from build123d import *

# Parameters (mm, degrees)
SKETCH1_R           = 9.525
SKETCH1_R_2         = 4.445
BOSS_EXTRUDE1_DEPTH = 3.048
SKETCH2_R           = 6.985
SKETCH2_R_2         = 4.445
BOSS_EXTRUDE2_DEPTH = 57.912
SKETCH3_R           = 9.525
SKETCH3_R_2         = 6.985
SKETCH3_R_3         = 4.445
BOSS_EXTRUDE3_DEPTH = 3.048


with BuildPart() as part:
    # Sketch1 → Boss-Extrude1 (new body)
    with BuildSketch(Plane(origin=(0, 0, 0), x_dir=(1, 0, 0), z_dir=(0, 1, 0))):
        with Locations(Location((0, 0, 0), (0, 0, 270))):  # turned: the seam where the file's is
            Circle(SKETCH1_R)
        with Locations(Location((0, 0, 0), (0, 0, 270))):  # turned: the seam where the file's is
            Circle(SKETCH1_R_2, mode=Mode.SUBTRACT)
    extrude(amount=BOSS_EXTRUDE1_DEPTH)

    # Sketch2 → Boss-Extrude2 (add)
    with BuildSketch(Plane(origin=(0, 3.048, 0), x_dir=(1, 0, 0), z_dir=(0, 1, 0))):
        with Locations(Location((0, 0, 0), (0, 0, 270))):  # turned: the seam where the file's is
            Circle(SKETCH2_R)
        with Locations(Location((0, 0, 0), (0, 0, 270))):  # turned: the seam where the file's is
            Circle(SKETCH2_R_2, mode=Mode.SUBTRACT)
    extrude(amount=BOSS_EXTRUDE2_DEPTH)

    # Sketch3 → Boss-Extrude3 (add)
    with BuildSketch(Plane(origin=(0, 60.96, 0), x_dir=(1, 0, 0), z_dir=(0, 1, 0))):
        with Locations(Location((0, 0, 0), (0, 0, 270))):  # turned: the seam where the file's is
            Circle(SKETCH3_R)
        with Locations(Location((0, 0, 0), (0, 0, 270))):  # turned: the seam where the file's is
            Circle(SKETCH3_R_2, mode=Mode.SUBTRACT)
        with Locations(Location((0, 0, 0), (0, 0, 270))):  # turned: the seam where the file's is
            Circle(SKETCH3_R_2)
        with Locations(Location((0, 0, 0), (0, 0, 270))):  # turned: the seam where the file's is
            Circle(SKETCH3_R_3, mode=Mode.SUBTRACT)
    extrude(amount=BOSS_EXTRUDE3_DEPTH)


solid = part.part
Could you check a few things on this model? Use its own coordinates, in mm. A direction names the side the tool comes from. Round coordinates to 2 decimals unless told otherwise and drop trailing zeros. Write each loop counter-clockwise with the first axis right and the second up, starting at its lowest first coordinate (ties: lowest second). Pieces come first, ordered by that corner, then holes. Notation, with made-up numbers: (86.25, 62.25) - (92.25, 62.25) arc R25 ccw to (92.25, 94.25) - close; hole circle Ø6 at (76.5, 31.25). An arc over 180 degrees is marked (long way). Put each result on its own line as item: value. Start each with the question number.
(1) Will these pins go through, and if not, where does the flat tip stop? pin 1 (5.5 mm diameter, centred on x = 2.5, z = -3.5, fed in from +Y); pin 2 (4 mm diameter, centred on y = 27, z = -1.5, fed in from +X) (3 decimals); pin 3 (6 mm diameter, centred on y = 49.5, z = 6, fed in from +X); pin 4 (1.5 mm diameter, centred on y = 41.5, z = -4, fed in from -X).
(2) For faces 1 (the flat face through (2.3, 0, 4.1)), 2 (the flat face through (7.1, 60.96, -0.8)), which set-ups out of +Z, -Z, +X, -X, +Y, -Y let a thin tool reach every point of the face, with its end or its side?
(3) I want a section at C-C, the plane y = 8.5. Please give me the cut outline in (x, z) (3 decimals), plus the area to 3 significant figures.
(4) I want a section at B-B, the plane x = 0. Please give me the cut outline in (y, z) (3 decimals).
(5) I need wall thicknesses on probe 1 along Y at (x, z) = (7.5, -1.5); probe 2 along X at (y, z) = (21, 0) (3 decimals); probe 3 along X at (y, z) = (21, 1.5). Which ranges of each line are inside material? Lowest first, please.
(6) I want a section at D-D, the plane x = -5.5. Please give me the cut outline in (y, z).
(7) I want a section at A-A, the plane z = 0. Please give me the cut outline in (x, y) (3 decimals), plus the area to 3 significant figures.
(8) Thinking about a two-plate mould opening in X: for faces 3 (the flat face through (2.3, 64.008, 4.1)), 4 (the cylindrical face through (-4.34, 31.56, -0.96)), 5 (the cylindrical face through (-5.796, 1.503, -7.559)), which applies, released by +X, released by -X, zero draft, split by the parting line, or undercut?
Here are the results:
1. pin 1: stops at y = 64.01
1. pin 2: stops at x = 6.985
1. pin 3: stops at x = 6.31
1. pin 4: stops at x = -6.18
2. face 1: +Z, -Z, +X, -X, -Y
2. face 2: none
3. outline: circle Ø13.97 at (0, 0); hole circle Ø8.89 at (0, 0)
3. area: 91.2 mm^2
4. outline: (0, -9.525) - (3.048, -9.525) - (3.048, -6.985) - (60.96, -6.985) - (60.96, -9.525) - (64.008, -9.525) - (64.008, -4.445) - (0, -4.445) - close; (0, 4.445) - (64.008, 4.445) - (64.008, 9.525) - (60.96, 9.525) - (60.96, 6.985) - (3.048, 6.985) - (3.048, 9.525) - (0, 9.525) - close
5. probe 1: y = 0 to 3.05, 60.96 to 64.01
5. probe 2: x = -6.985 to -4.445, 4.445 to 6.985
5. probe 3: x = -6.82 to -4.18, 4.18 to 6.82
6. outline: (0, -7.78) - (3.05, -7.78) - (3.05, -4.31) - (60.96, -4.31) - (60.96, -7.78) - (64.01, -7.78) - (64.01, 7.78) - (60.96, 7.78) - (60.96, 4.31) - (3.05, 4.31) - (3.05, 7.78) - (0, 7.78) - close
7. outline: (-9.525, 0) - (-4.445, 0) - (-4.445, 64.008) - (-9.525, 64.008) - (-9.525, 60.96) - (-6.985, 60.96) - (-6.985, 3.048) - (-9.525, 3.048) - close; (4.445, 0) - (9.525, 0) - (9.525, 3.048) - (6.985, 3.048) - (6.985, 60.96) - (9.525, 60.96) - (9.525, 64.008) - (4.445, 64.008) - close
7. area: 356 mm^2
8. face 3: zero draft
8. face 4: undercut
8. face 5: split by the parting line
